Here's how the part is built. I have some questions about the finished solid (model axes, mm). A direction names the side the tool comes from. Coordinates: 2 decimals unless noted, no trailing zeros. Write each loop counter-clockwise with the first axis right and the second up, starting at its lowest first coordinate (ties: lowest second). Pieces come first, ordered by that corner, then holes.
Item 1: I want a section at B-B (z = 8). Please give me the cut outline in (x, y).
Item 2: For faces 5 (the face through (-1, 5, 15)), 6 (the face through (100, -1, 3)), which set-ups out of +Z, -Z, +X, -X, +Y, -Y let a thin tool reach every point of the face, with its end or its side?
Item 3: I want a section at A-A (x = 36). Please give me the cut outline in (y, z), and give its area (3 significant figures).
Item 4: If we mould it in two halves opening along Y, with no side actions, what happens to faces 1 (the face through (-1, -5, 15)), 2 (the face through (-1, 0, 5)), 3 (the face through (-1, 28, 20)), 4 (the face through (-1, -50, 10))? For each: pulls with the +Y half, pulls with the -Y half, needs draft (parallel to the pull), parting line crosses it, or undercut.
Item 5: I want a section at C-C (y = 0). Please give me the cut outline in (x, z).
Item 6: Please list where these lines run through material, in increasing order: line 1 (Y direction, x = 85.5, z = 15.25); line 2 (Y direction, x = -14, z = 8); line 3 (Z direction, x = 56.5, y = 4).
from build123d import *

# Parameters (mm, degrees)
SKETCH_1_W          = 200
SKETCH_1_H          = 100
EXTRUDE_1_DEPTH     = 20
CUT_EXTRUDE_1_DEPTH = 201


with BuildPart() as part:
    # 草图1 → 凸台-拉伸1 (new body)
    with BuildSketch(Plane.XY):
        Rectangle(SKETCH_1_W, SKETCH_1_H)
    extrude(amount=EXTRUDE_1_DEPTH)

    # 草图2 → 切除-拉伸1 (cut, through all)
    with BuildSketch(Plane.ZY.offset(100)):
        with BuildLine():
            Line((10, -5), (20, -5))
            Line((20, -5), (20, 5))
            Line((20, 5), (10, 5))
            ThreePointArc((10, 5), (5, 0), (10, -5))
        make_face()
    extrude(amount=-CUT_EXTRUDE_1_DEPTH, mode=Mode.SUBTRACT)


solid = part.part
Answer:
1. outline: (-100, -50) - (100, -50) - (100, -4.58) - (-100, -4.58) - close; (-100, 4.58) - (100, 4.58) - (100, 50) - (-100, 50) - close
2. face 5: +Z, +X, -X
2. face 6: +Z, -Z, +X, +Y, -Y
3. outline: (-50, 0) - (50, 0) - (50, 20) - (5, 20) - (5, 10) arc R5 cw to (-5, 10) - (-5, 20) - (-50, 20) - close
3. area: 1,860 mm2
4. face 1: undercut
4. face 2: undercut
4. face 3: needs draft
4. face 4: pulls with the -Y half
5. outline: (-100, 0) - (100, 0) - (100, 5) - (-100, 5) - close
6. line 1: y = -50 to -5, 5 to 50
6. line 2: y = -50 to -4.58, 4.58 to 50
6. line 3: z = 0 to 7
